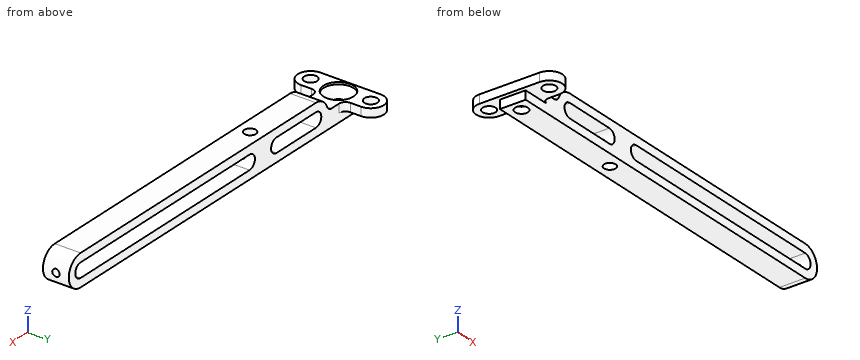
```python
from build123d import *

# Parameters (mm, degrees)
F1_DEPTH       = 3
F3_DEPTH       = 6
F5_DEPTH       = 2
F6_R           = 3.5
F7_DEPTH       = 0.5
F9_D           = 3
F9_CSINK_D     = 7
F9_CSINK_ANGLE = 90
F10_D          = 3
F11_R          = 1.5
F14_R          = 0.85
F15_DEPTH      = 63.7357865376
F17_D          = 2.7
F18_SCALE      = 1.02


with BuildPart() as f1:
    # F0 (on Front) → F1 (new body, symmetric)
    with BuildSketch(Plane.XZ):
        with BuildLine():
            ThreePointArc((0, 3.65), (-3.65, 0), (0, -3.65))
            Line((0, -3.65), (72.7, -3.65))
            ThreePointArc((72.7, -3.65), (76.35, 0), (72.7, 3.65))
            Line((72.7, 3.65), (0, 3.65))
        make_face()
        with BuildLine():
            Line((12.2, -1.65), (0, -1.65))
            ThreePointArc((0, -1.65), (-1.65, 0), (0, 1.65))
            Line((0, 1.65), (12.2, 1.65))
            ThreePointArc((12.2, 1.65), (13.85, 0), (12.2, -1.65))
        make_face(mode=Mode.SUBTRACT)
        with BuildLine():
            Line((20.5, 1.65), (72.7, 1.65))
            ThreePointArc((72.7, 1.65), (74.35, 0), (72.7, -1.65))
            Line((72.7, -1.65), (20.5, -1.65))
            ThreePointArc((20.5, -1.65), (18.85, 0), (20.5, 1.65))
        make_face(mode=Mode.SUBTRACT)
    extrude(amount=F1_DEPTH, both=True)

    # F2 (on face) → F3 (join, through all)
    with BuildSketch(Plane.XZ.offset(3)):
        with BuildLine():
            Line((-13.65, -3.65), (0, -3.65))
            ThreePointArc((0, -3.65), (-2.7018512172, -2.4540782384), (-3.6331804249, 0.35))
            Line((-3.6331804249, 0.35), (-13.65, 0.35))
            Line((-13.65, 0.35), (-13.65, -3.65))
        make_face()
    extrude(amount=-F3_DEPTH)

    # F4 (on face) → F5 (join)
    with BuildSketch(Plane.XY.offset(0.35)):
        with BuildLine():
            ThreePointArc((-14.65, -7), (-11.65, -10), (-8.65, -7))
            Line((-8.65, -7), (-8.65, 7))
            ThreePointArc((-8.65, 7), (-11.65, 10), (-14.65, 7))
            Line((-14.65, 7), (-14.65, -7))
        make_face()
    extrude(amount=-F5_DEPTH)

    # F6 (on face) → F7 (cut)
    with BuildSketch(Plane.XY.offset(0.35)):
        with Locations((-10.95, 0)):
            Circle(F6_R)
    extrude(amount=-F7_DEPTH, mode=Mode.SUBTRACT)

    # F9 (through all)
    with Locations(Plane.XY.offset(-0.15)):
        with Locations((-10.95, 0)):
            CounterSinkHole(F9_D / 2, F9_CSINK_D / 2, counter_sink_angle=F9_CSINK_ANGLE)

    # F10 (through all)
    with Locations(Plane.XY.offset(0.35)):
        with Locations((-11.65, 7), (-11.65, -7)):
            Hole(F10_D / 2)

    # F11
    f11_edges = [f1.edges().sort_by_distance(p)[0] for p in [
        (-8.65, -3, -0.65),
        (-8.65, 3, -0.65),
        (-3.63318, 0, 0.35),
    ]]
    fillet(f11_edges, radius=F11_R)

    # F14 (on plane+point) → F15 (cut, up to face)
    with BuildSketch(Plane.YZ.offset(76.35)):
        Circle(F14_R)
    extrude(amount=-F15_DEPTH, mode=Mode.SUBTRACT)

    # F17 (through all)
    with Locations(Plane.XY.offset(3.65)):
        with Locations((16.35, 0)):
            Hole(F17_D / 2)


with BuildPart() as f1_1:
    # F18: moved
    add(f1.part.scale(F18_SCALE))


solid = f1_1.part
```
Part model, mm, in its own coordinate system. Round coordinates to 2 decimals unless told otherwise and drop trailing zeros. Order: outer loops, then holes, each group sorted by start corner. A loop starts at its lowest first (then second) coordinate and runs counter-clockwise, first axis right, second up. Notation, with made-up numbers: M 13.5,78.5 L 45.5,78.5 A30 ccw 45.5,104.5 Z; hole C 39.25,-29.75 d3. An arc over 180 degrees is marked long. Put each result on its own line as item: value. Start each with the question number.
1. Drill centre lines: probe 1 along Z at (x, y) = (53, 1); probe 2 along Z at (x, y) = (15.2, 0); probe 3 along Y at (x, z) = (41, -2.25). Where is each one in solid material? Low to high. Write a range as [from, to].
2. Slice it at A-A on x = 39. List the corners of the cut face in (y, z).
3. Drop flat-ended pins along their axis: pin 1 (5 mm diameter, centred on x = -11.883, y = 7.14, fed in from -Z); pin 2 (2 mm diameter, centred on y = -6, z = -0.5, fed in from +X); pin 3 (2 mm diameter, centred on x = 13.5, z = 3, fed in from -Y). Give the stop position or say it passes through.
4. Slice it at B-B on z = 2.75. List the corners of the cut face in (x, y), then the cut area to 3 significant figures.
Findings:
1. probe 1: [-3.72, -1.68], [1.68, 3.72]
1. probe 2: [-3.72, -0.87], [0.87, 3.72]
1. probe 3: [-3.06, 3.06]
2. outline: M -3.06,-3.72 L 3.06,-3.72 L 3.06,-1.68 L -3.06,-1.68 Z; M -3.06,1.68 L 3.06,1.68 L 3.06,3.72 L -3.06,3.72 Z
3. pin 1: z = -1.68
3. pin 2: x = -8.82
3. pin 3: y = -3.06
4. outline: M -2.51,-3.06 L 76.66,-3.06 L 76.66,3.06 L -2.51,3.06 Z; hole C 16.68,0 d2.75
4. area: 479 mm2
